Design review of the part built by this model. Coordinates are the model's own, in mm. A direction names the side the tool comes from. Give positions to 0.01 mm unless a question says otherwise; leave off trailing zeros. Loops run counter-clockwise (first coordinate to the right, second up) from the corner with the lowest first, then second, coordinate; pieces in that order, holes last. Notation, with made-up numbers: (37, 88.5) - (68, 88.5) arc R30 cw to (68, 124.5) - close; hole circle Ø6 at (54, 27). An arc over 180 degrees is marked (long way). Write each question's results on one line, items separated by ' | '.
Autodesk Inventor part; units mm, degrees
ref_plane "YZ Plane" through (0, 0, 0) normal (1, 0, 0) x (0, 1, 0)
ref_plane "XZ Plane" through (0, 0, 0) normal (0, 1, 0) x (-1, 0, 0)
ref_plane "XY Plane" through (0, 0, 0) normal (0, 0, 1) x (1, 0, 0)
sketch "Sketch1" plane through (0, 0, 0) normal (0, 0, 1) x (1, 0, 0)
  circle A0 centre (0, 0) radius 11
  circle A1 centre (0, 0) radius 8 construction
  line L0 (0, 0) -> (0, 8) construction
  circle A2 centre (0, 8) radius 1.75
  line L1 (0, 0) -> (-8, 0) construction
  circle A3 centre (-8, 0) radius 1.75
  line L2 (0, 0) -> (0, -8) construction
  circle A4 centre (0, -8) radius 1.75
  line L3 (0, 0) -> (8, 0) construction
  circle A5 centre (8, 0) radius 1.75
  dimension "d1" = 16
  dimension "d0" = 22
  dimension "d2" = 3.5
  dimension "d5" = 360
extrude "Extrusion1" add sketch "Sketch1" along normal blind 5
sketch "Sketch2" plane through (0, 0, 5) normal (0, 0, 1) x (1, 0, 0)
  circle A0 centre (0, 0) radius 5.1
  dimension "d10" = 10.2
sketch "Sketch3" plane through (0, 0, 0) normal (0, 0, -1) x (-1, 0, 0)
  point P0 (0, 0)
extrude "Extrusion2" add sketch "Sketch2" along normal blind 1.5
sketch "Sketch4" plane through (0, 0, 0) normal (0, 0, -1) x (-1, 0, 0)
  circle A0 centre (0, 0) radius 5.1
  dimension "d13" = 10.2
extrude "Extrusion3" add sketch "Sketch4" along normal blind 10
sketch "Sketch5" plane through (0, 0, 6.5) normal (0, 0, 1) x (1, 0, 0)
  circle A0 centre (0, 0) radius 4.1
  dimension "d16" = 8.2
extrude "Extrusion4" cut sketch "Sketch5" against normal blind 19.5
thread "Thread1"
fillet "Fillet1" radius 0.5 2 edges at (-11, 0, 5) (-11, 0, 0)
properties part number "LeadNut"
(1) Take a section at A-A on x = 0. Give the boundary of the cut face in (y, z), plus the area to 3 significant figures.
Answers below:
outline: (-11, 0.5) arc R0.5 ccw to (-10.5, 0) - (-9.75, 0) - (-9.75, 5) - (-10.5, 5) arc R0.5 ccw to (-11, 4.5) - close; (-6.25, 0) - (-5.1, 0) - (-5.1, -10) - (-4.1, -10) - (-4.1, 6.5) - (-5.1, 6.5) - (-5.1, 5) - (-6.25, 5) - close; (4.1, -10) - (5.1, -10) - (5.1, 0) - (6.25, 0) - (6.25, 5) - (5.1, 5) - (5.1, 6.5) - (4.1, 6.5) - close; (9.75, 0) - (10.5, 0) arc R0.5 ccw to (11, 0.5) - (11, 4.5) arc R0.5 ccw to (10.5, 5) - (9.75, 5) - close | area: 56.8 mm2
(2) Take a section at D-D on z = -9. Give the boundary of the cut face in (x, y).
Answers below:
outline: circle Ø10.2 at (0, 0); hole circle Ø8.2 at (0, 0)
(3) Tool access review of faces 1 (the cylindrical face through (-0.228, -9.735, 2.465)), 2 (the cylindrical face through (-2.4, 4.5, -4.9)), 3 (the cylindrical face through (2.4, 4.5, 5.7)): name each direction out of +Z, -Z, +X, -X, +Y, -Y from which nothing blocks a thin tool from reaching the whole face with its end or side.
Answers below:
face 1: +Z, -Z | face 2: -Z | face 3: +Z
(4) Take a section at C-C on z = 1. Give the boundary of the cut face in (x, y), plus the area to 3 significant figures.
Answers below:
outline: circle Ø22 at (0, 0); hole circle Ø3.5 at (-8, 0); hole circle Ø8.2 at (0, 0); hole circle Ø3.5 at (0, -8); hole circle Ø3.5 at (0, 8); hole circle Ø3.5 at (8, 0) | area: 289 mm2
(5) Insertion check: P1, Ø5.5, axis at x = 8, y = 0, coming from the +Z side; P2, Ø4, axis at x = -6, y = -8.5, coming from the -Z side; P3, Ø4, axis at x = -7, z = 4.5, coming from the -Y side. Each pin has a flat end and moves straight along its axis. Give the tip position at first contact, or say it passes through.
Answers below:
P1: z = 5 | P2: z = 0 | P3: y = -9.8
(6) Draft analysis for pull direction X (two halves, no side actions). For faces 4 (the cylindrical face through (-2.38, 10.74, 2.47)), 5 (the cylindrical face through (-0.534, 4.065, -1.634)), 6 (the flat face through (5, 2, 0)), state which applies: pulls with the +X half, pulls with the -X half, needs draft (parallel to the pull), parting line crosses it, or undercut.
Answers below:
face 4: parting line crosses it | face 5: undercut | face 6: needs draft
(7) Wall thickness on line 1 along Y through (x, z) = (0, 3.55); line 2 along Y through (x, z) = (0, -5.5); line 3 along Z through (x, y) = (7.5, -4.5): over which ranges is each line inside the solid? List them lowest first. Write a range as from..to.
Answers below:
line 1: -11..-9.75, -6.25..-4.1, 4.1..6.25, 9.75..11 | line 2: -5.1..-4.1, 4.1..5.1 | line 3: 0..5
